For this review, take the finished solid that the model builds, in its own axes (mm). Face numbers are marked on the shaded views. A direction names the side the tool comes from. Give positions to 0.01 mm unless a question says otherwise; leave off trailing zeros. Write each loop counter-clockwise with the first axis right and the second up, starting at its lowest first coordinate (ties: lowest second). Pieces come first, ordered by that corner, then holes.
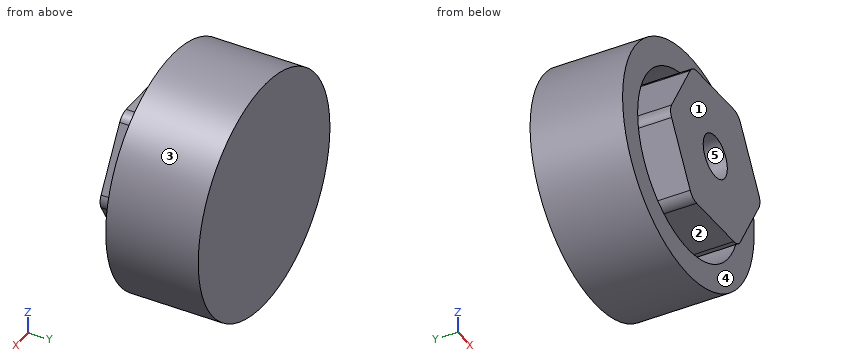
Autodesk Inventor part; units mm, degrees
ref_plane "YZ Plane" through (0, 0, 0) normal (1, 0, 0) x (0, 1, 0)
ref_plane "XZ Plane" through (0, 0, 0) normal (0, 1, 0) x (-1, 0, 0)
ref_plane "XY Plane" through (0, 0, 0) normal (0, 0, 1) x (1, 0, 0)
sketch "Sketch1" plane through (0, 0, 0) normal (0, 1, 0) x (-1, 0, 0)
  line L0 (-8.75, 22.75) -> (8.75, 22.75)
  line L1 (8.75, 22.75) -> (8.75, -22.75)
  line L2 (8.75, -22.75) -> (-8.75, -22.75)
  line L3 (-8.75, -22.75) -> (-8.75, 22.75)
  line L4 (-8.75, 22.75) -> (8.75, -22.75) construction
  line L5 (8.75, 22.75) -> (-8.75, -22.75) construction
  line L6 (-1.6021, -2.775) -> (-3.2043, 0)
  line L7 (-3.2043, 0) -> (-1.6021, 2.775)
  line L8 (-1.6021, 2.775) -> (1.6021, 2.775)
  line L9 (1.6021, 2.775) -> (3.2043, 0)
  line L10 (3.2043, 0) -> (1.6021, -2.775)
  line L11 (1.6021, -2.775) -> (-1.6021, -2.775)
  line L12 (6.091, 0) -> (3.0455, 5.275)
  line L13 (3.0455, 5.275) -> (-3.0455, 5.275)
  line L14 (-3.0455, 5.275) -> (-6.091, 0)
  line L15 (-6.091, 0) -> (-3.0455, -5.275)
  line L16 (-3.0455, -5.275) -> (3.0455, -5.275)
  line L17 (3.0455, -5.275) -> (6.091, 0)
  line L18 (6.75, -20.75) -> (6.75, 20.75)
  line L19 (6.75, 20.75) -> (-6.75, 20.75)
  line L20 (-6.75, 20.75) -> (-6.75, -20.75)
  line L21 (-6.75, -20.75) -> (6.75, -20.75)
  circle A0 centre (0, 0) radius 1.6
  circle A1 centre (0, 0) radius 8.75
  circle A2 centre (0, 0) radius 6.75
  dimension "d0" = 17.5
  dimension "d1" = 45.5
  dimension "d2" = 5.55
  dimension "d8" = 2.5
  dimension "d9" = 2
  dimension "d11" = 3.2
  dimension "d14" = 17.5
  dimension "d15" = 2
extrude "Extrusion1" add sketch "Sketch1" along normal blind 6.9 contours A1 L20 | A1 L18 | A1 L18 A2 L20 | L20 A2 L18 A1 | A2 | L6 L7 L8 L9 L10 L11 | L17 L16 L15 L14 L13 L12 | A0
extrude "Extrusion5" add sketch "Sketch1" against normal blind 2 contours L6 L7 L8 L9 L10 L11 | L17 L16 L15 L14 L13 L12
extrude "Extrusion2" cut sketch "Sketch1" along normal blind 4 contours A2 | L6 L7 L8 L9 L10 L11 | A0
fillet "Fillet1" radius 1 6 edges at (6.091, 1, 0) (-3.0455, 1, 5.275) (3.0455, 1, -5.275) (-3.0455, 1, -5.275) (-6.091, 1, 0) (3.0455, 1, 5.275)
fillet "Fillet2" [suppressed]
equation "\"d14\" = d0"
properties part number "Solenoid Shield"
(1) The part is to be moulded in two halves that separate along Z. For the marked faces 3, 4 and 5, say which applies: +Z half, -Z half, draft (parallel to the pull), parting line (faces both ways), or undercut.
(2) Clearance check with flat-ended pins moving along their axes: pin 1 Ø4 at (y, z) = (3.5, 6) entering from -X; pin 2 Ø1 at (x, z) = (5, 4) entering from -Y; pin 3 Ø1.5 at (x, y) = (4.5, 6) entering from -Z. State where each tip first meets the part, or that it passes through.
(3) Tool access review of the marked faces 1 and 2: name each direction out of +Z, -Z, +X, -X, +Y, -Y from which nothing blocks a thin tool from reaching the whole face with its end or side.
(4) We need section D-D (x = 2.25). Write out the cut boundary in (y, z) (3 decimals).
(5) We need section B-B (x = 0). Write out the cut boundary in (y, z) (3 decimals), and give its area (3 significant figures).
(6) For L1, parallel to Z at x = 0, y = 2.25 (3 decimals); L2, parallel to Z at x = 0, y = -1.25 (3 decimals); L3, parallel to Z at x = -3, y = 3, list the stretches that pass through material, from the lowest coordinate up.
(7) We need section A-A (y = 2.25). Write out the cut boundary in (x, z) (3 decimals).
(8) We need section C-C (z = 4). Write out the cut boundary in (x, y).
The answers:
1. face 3: parting line
1. face 4: draft
1. face 5: undercut
2. pin 1: stops at x = -7.78
2. pin 2: stops at y = 0
2. pin 3: stops at z = -7.91
3. face 1: +Z, -Z, +X, -X, -Y
3. face 2: -Y
4. outline: (-2, -5.275) - (4, -5.275) - (4, -6.364) - (0, -6.364) - (0, -8.456) - (6.9, -8.456) - (6.9, 8.456) - (0, 8.456) - (0, 6.364) - (4, 6.364) - (4, 5.275) - (-2, 5.275) - close; hole (0, -1.653) - (4, -1.653) - (4, 1.653) - (0, 1.653) - close
5. outline: (-2, -5.275) - (4, -5.275) - (4, -6.75) - (0, -6.75) - (0, -8.75) - (6.9, -8.75) - (6.9, 8.75) - (0, 8.75) - (0, 6.75) - (4, 6.75) - (4, 5.275) - (-2, 5.275) - (-2, 1.6) - (0, 1.6) - (0, 2.775) - (4, 2.775) - (4, -2.775) - (0, -2.775) - (0, -1.6) - (-2, -1.6) - close
5. area: 101 mm2
6. L1: z = -8.75 to -6.75, -5.275 to -2.775, 2.775 to 5.275, 6.75 to 8.75
6. L2: z = -5.275 to -1.6, 1.6 to 5.275
6. L3: z = -8.22 to -6.05, -5.12 to -0.35, 0.35 to 5.12, 6.05 to 8.22
7. outline: circle Ø17.5 at (0, 0); (-5.802, -0.5) - (-3.334, -4.775) arc R1 ccw to (-2.468, -5.275) - (2.468, -5.275) arc R1 ccw to (3.334, -4.775) - (5.802, -0.5) arc R1 ccw to (5.802, 0.5) - (3.334, 4.775) arc R1 ccw to (2.468, 5.275) - (-2.468, 5.275) arc R1 ccw to (-3.334, 4.775) - (-5.802, 0.5) arc R1 ccw to start; hole circle Ø13.5 at (0, 0); hole (-3.204, 0) - (-1.602, -2.775) - (1.602, -2.775) - (3.204, 0) - (1.602, 2.775) - (-1.602, 2.775) - close
8. outline: (-7.78, 0) - (-5.44, 0) - (-5.44, 4) - (-3.78, 4) - (-3.78, -2) - (3.78, -2) - (3.78, 4) - (5.44, 4) - (5.44, 0) - (7.78, 0) - (7.78, 6.9) - (-7.78, 6.9) - close
